Design review of the part built by this model. Coordinates are the model's own, in mm. A direction names the side the tool comes from. Coordinates: 2 decimals unless noted, no trailing zeros. Loops run counter-clockwise (first coordinate to the right, second up) from the corner with the lowest first, then second, coordinate; pieces in that order, holes last.
Q1. Add section A-A on z = 21.5. Give the boundary of the cut face in (x, y), and give its area (3 significant figures).
Q2. Wall thickness on probe 1 along Y at (x, z) = (-14.5, -4); probe 2 along Y at (x, z) = (-21.5, 26.5); probe 3 along X at (y, z) = (23, 14.5): over which ranges is each line inside the solid? List them lowest first.
Q3. Machinability: for faces 1 (the face through (-14.6, 20.8, 0)), 2 (the face through (-23.244, 20.051, -6.261)), 3 (the face through (-23, 21, 0)), which of the approach directions +Z, -Z, +X, -X, +Y, -Y give a long, thin tool a straight path to every point of the face, cutting with its end or side? Answer none if there is none.
Q4. For P1, Ø1, axis at x = -21.5, z = 8, coming from the -Y side, flat-tipped, find the tip position at first contact; note if it passes through.
Q5. Add section B-B on x = -20. Give the boundary of the cut face in (y, z), and give its area (3 significant figures).
Q6. Add section C-C on x = -17.5. Give the boundary of the cut face in (y, z).
Autodesk Inventor part; units mm, degrees
ref_plane "YZ Plane" through (0, 0, 0) normal (1, 0, 0) x (0, 1, 0)
ref_plane "XZ Plane" through (0, 0, 0) normal (0, 1, 0) x (-1, 0, 0)
ref_plane "XY Plane" through (0, 0, 0) normal (0, 0, 1) x (1, 0, 0)
sketch "Sketch1" plane through (0, 0, 0) normal (0, 0, 1) x (1, 0, 0)
  line L0 (-16.4487, 14.1051) -> (-9.6381, 18.058)
  line L1 (-16.4487, 14.1051) -> (-18.8393, 18.2241)
  line L2 (-18.8393, 12.7176) -> (-23.6081, 15.4709)
  line L3 (-23.6081, 15.4709) -> (-23.6081, 20.9774)
  line L4 (-23.6081, 20.9774) -> (-18.8393, 23.7306)
  line L5 (-18.8393, 23.7306) -> (-14.0705, 20.9774)
  line L6 (-14.0705, 20.9774) -> (-14.0705, 15.4709)
  line L7 (-14.0705, 15.4709) -> (-18.8393, 12.7176)
  dimension "d5" = 4.7625
extrude "Extrusion1" add sketch "Sketch1" along normal blind 50.8
sketch "Sketch3" plane through (0, 0, 0) normal (0, 0, -1) x (-1, 0, 0)
  line L0 (23.6081, 15.4709) -> (18.8393, 12.7176)
  line L1 (18.8393, 12.7176) -> (18.8393, 18.2241)
  circle A0 centre (18.8393, 18.2241) radius 4.7688
  point P0 (0, 0)
extrude "Extrusion3" add sketch "Sketch3" along normal blind 12.7 contours A0
properties part number "Sanded Hex Rod"
Entries:
1. outline: (-23.61, 15.47) - (-18.84, 12.72) - (-14.07, 15.47) - (-14.07, 20.98) - (-18.84, 23.73) - (-23.61, 20.98) - close
1. area: 78.8 mm2
2. probe 1: y = 16.25 to 20.2
2. probe 2: y = 14.25 to 22.19
2. probe 3: x = -20.1 to -17.57
3. face 1: -Z, +X, +Y
3. face 2: -Z
3. face 3: -Z, -X, +Y
4. P1: stops at y = 13.97
5. outline: (13.39, 0) - (13.6, 0) - (13.6, -12.7) - (22.85, -12.7) - (22.85, 0) - (23.06, 0) - (23.06, 50.8) - (13.39, 50.8) - close
5. area: 609 mm2
6. outline: (13.49, 0) - (13.65, 0) - (13.65, -12.7) - (22.8, -12.7) - (22.8, 0) - (22.96, 0) - (22.96, 50.8) - (13.49, 50.8) - close
